from build123d import *

# Parameters (mm, degrees)
F0_R     = 2.9695482625
F1_DEPTH = 1
F4_DEPTH = 27.3


with BuildPart() as f1:
    # F0 (on Top) → F1 (new body, symmetric)
    with BuildSketch(Plane.XY):
        Polygon((12.3607597711, -55.2147076325), (16.7780640493, -50.0796457731), (16.7780640493, -27.9147076325), (18.8081849192, -27.9147076325), (19.2885116058, -27.4970311455), (19.5391171796, -27.2673100327), (19.5391171796, -26.9958199979), (19.5391171796, -26.7243331464), (19.5391171796, -26.2857721985), (18.0981371197, -24.0512096784), (18.0981371197, -23.7379539049), (18.1399044501, -23.5500001224), (18.3487426936, -23.3202774179), (18.5784638064, -22.9443698531), (19.601768971, -22.2134375926), (20.6041896746, -21.3780878021), (21.3977721348, -20.5636208809), (22.3375426387, -19.3732463948), (23.0475904382, -18.475244813), (23.3817306727, -17.7234280915), (23.7785211069, -17.1386838748), (23.94559202, -16.4704034057), (24.1126613415, -16.0736113798), (24.3107286721, -15.2382599976), (24.3107286721, -14.5422572011), (24.4967819861, -13.5003595977), (24.4967819861, -12.1979863997), (24.1618857025, -10.5979288543), (23.6781480411, -8.6629758211), (23.0083570657, -6.9884967909), (22.1897215291, -5.723335529), (20.9989809561, -4.4581734713), (19.5105560358, -3.1930120105), (17.5383918623, -2.0394821799), (15.7894929391, -1.3696908066), (14.5987523661, -1.0832198235), (10.7237476301, -1.0832198235), (9.7613685895, -1.4441120924), (8.2729436691, -2.0022716365), (6.9333601266, -2.6348524664), (5.3333029791, -3.7139610111), (4.3658260647, -4.6070164409), (3.5844024642, -5.5000718706), (2.8029794606, -6.6908124435), (2.0587666025, -8.0676063305), (1.7238711148, -9.1467142784), (1.4261855736, -10.0769800525), (1.3145539433, -10.8956139975), (1.3145539433, -11.6398272535), (1.3145539433, -15.3981014905), (1.6272404915, -15.9329066809), (2.0135845171, -16.8460833601), (2.6106608878, -18.0402364995), (3.4887149126, -19.5153676908), (4.1560359953, -20.498788485), (4.7882354184, -21.2714753424), (5.7716558147, -22.079285849), (6.8604427815, -22.851974298), (7.2781184726, -23.1652316632), (7.6540260375, -23.4993718978), (7.9046308155, -23.7917448019), (8.1761200545, -24.0632332451), (8.5280640493, -24.418256349), (8.5280640493, -24.8359328359), (8.5280640493, -25.2878464051), (8.5280640493, -50.8238519687), (11.0211762286, -54.6565492822), (11.4304932011, -55.2147076325), (11.8025998291, -55.2147076325), align=None)
        with Locations((12.8210000694, -8.8269943371)):
            Circle(F0_R, mode=Mode.SUBTRACT)
    extrude(amount=F1_DEPTH, both=True)

    # F3 (on offset) → F4 (cut)
    with BuildSketch(Plane.XZ.offset(55.2147076325)):
        Polygon((17.2618441284, 1.6106185503), (7.4076484889, 1.6106185503), (7.2416369803, -2.3955139332), (17.2618441284, -2.3955139332), align=None)
        Polygon((8.4565682159, -1), (8.5280640493, 1), (11.0793640826, 1), (11.3692851097, 0.5361280251), (11.6591977943, 0.0142720533), (11.9201283872, -0.3336319279), (12.3550099279, -0.623552955), (12.9348519822, -0.7105284289), (13.4567048255, -0.7105284289), (13.804606721, -0.3626244477), (14.1235181824, -0.0437119435), (14.4134392095, 0.2751995178), (14.6743698024, 0.594112022), (14.7975728908, 0.7176237855), (15.1462589881, 0.7176237855), (15.6111821269, 0.6272226434), (16.0244438949, 0.5368215013), (16.3473055636, 0.4205907166), (16.6830815322, 0.3301895745), (16.7993144025, -0.2122183209), (16.6828928362, -0.237166359), (16.4764527338, -0.1089018361), (16.2181625646, 0.0460718483), (15.9082151958, 0.1752158901), (15.5853535271, 0.1752158901), (15.1333446882, 0.1752158901), (14.9267158898, 0.0719004481), (14.7071727916, -0.0443292938), (14.5651071501, -0.2509612206), (14.3713926517, -0.509250347), (14.2164210529, -0.7546251735), (14.0485268117, -0.9612571003), (13.9193838127, -1.0516582424), (11.9434709008, -1.0516582424), (11.6076991035, -0.5350799896), (11.2590046637, 0.084814748), (10.8586530244, 0.2914466748), (10.5616241267, 0.4593346591), (10.2258439869, 0.4593346591), (9.9029864894, 0.4593346591), (9.6705290913, 0.3301895745), (9.386406151, 0.1752158901), (9.1539487529, -0.0055863941), (9.1539487529, -0.2251326208), (8.9989771541, -0.5609085894), (8.8439972128, -0.7804548161), (8.8439972128, -0.9870857001), (8.6373684144, -1), align=None, mode=Mode.SUBTRACT)
    extrude(amount=-F4_DEPTH, mode=Mode.SUBTRACT)


solid = f1.part
Source: CAD feature listing. Evaluate the final solid. Frame: model axes, mm. Coordinates: 2 decimals unless noted, no trailing zeros. Order: outer loops, then holes, each group sorted by start corner. A loop starts at its lowest first (then second) coordinate and runs counter-clockwise, first axis right, second up. Notation, with made-up numbers: M -34.75,48 L -5.75,48 A10 ccw -5.75,65 Z; hole C 32,66.25 d2. An arc over 180 degrees is marked long. Write each question's results on one line, items separated by ' | '. Start each with the question number.
Item 1: Draft query along Y for faces 1 (the face through (19.083, -22.584, 0.014)), 2 (the face through (24.402, -14.029, 0.014)), 3 (the face through (1.315, -13, 0)). Return one class per face: pulls with the +Y half, pulls with the -Y half, needs draft (parallel to the pull), parting line crosses it, or undercut.
Item 2: Cut plane A-A (y = -20). Return loops of the section in (x, z).
Item 3: First-contact query: pin 1 Ø0.6 at (x, y) = (13, -38) entering from +Z; pin 2 Ø0.7 at (x, y) = (10, -44.5) entering from -Z. Flat tips, straight axial feed; report the tip coordinate or a pass-through.
Item 4: Line query: probe 1 along X at (y, z) = (-50.5, 0.3); probe 2 along X at (y, z) = (-43, -0.3); probe 3 along X at (y, z) = (-27, -0.1). Output: solid intervals per line, ascending.
Checked values:
1) face 1: undercut | face 2: pulls with the -Y half | face 3: needs draft
2) outline: M 3.82,-1 L 21.84,-1 L 21.84,1 L 3.82,1 Z
3) pin 1: stops at z = -0.68 | pin 2: stops at z = 0.32
4) probe 1: x = 8.53 to 9.62, 10.84 to 11.5, 14.43 to 16.42 | probe 2: x = 8.53 to 9.12, 11.48 to 11.89, 13.87 to 14.53 | probe 3: x = 8.53 to 19.54
